The model under review builds one solid part; all positions refer to its coordinate system, in mm. A direction names the side the tool comes from. Round coordinates to 2 decimals unless told otherwise and drop trailing zeros. Write each loop counter-clockwise with the first axis right and the second up, starting at its lowest first coordinate (ties: lowest second). Pieces come first, ordered by that corner, then holes. Notation, with made-up numbers: (68, 29.5) -> (125, 29.5) arc R24 ccw to (125, 41.5) -> close; hole circle Ø6 at (76, -5). An arc over 180 degrees is marked (long way). Return JSON: item names as keys, results as strings. Group by question number.
1. Take a section at B-B, the plane x = -7.5. Write out the cut boundary in (y, z).
2. For line 1 along Z through (x, y) = (-7.3, -10.2); line 2 along X through (y, z) = (-70, 0.5); line 3 along Y through (x, z) = (-8.8, -10), list the stretches that pass through material, from the lowest coordinate up. Write a range as from..to.
3. Take a section at C-C, the plane y = -36. Write out the cut boundary in (x, z).
4. Clearance check with a flat-ended pin moving along its axis: P1, Ø14.5, axis at y = -78, z = 6.5, coming from the +X side. State where the tip first meets the part, or that it passes through.
5. Mouldability with a two-part tool opening along Y and no side actions: class faces 4 (the flat face through (-9.15, -127.44, 2.59)), 5 (the flat face through (-8, 0, -1)), 6 (the flat face through (-9, -50, 11.847)), 7 (the cylindrical face through (-8.083, -9.658, 3.207)) as pulls with the +Y half, pulls with the -Y half, needs draft (parallel to the pull), parting line crosses it, or undercut.
6. Take a section at A-A, the plane y = -10.2. Write out the cut boundary in (x, z).
7. Tool access review of faces 1 (the flat face through (-9.168, -66.634, -7.842)), 2 (the flat face through (-8, -16, -14.153)), 3 (the flat face through (-8.661, -81, 5)): name each direction out of +Z, -Z, +X, -X, +Y, -Y from which nothing blocks a thin tool from reaching the whole face with its end or side.
from build123d import *

# Parameters (mm, degrees)
F1_DEPTH = 31.5
F2_DEPTH = 131.5
F6_DEPTH = 25
F7_D     = 5
F7_DEPTH = 300
F7_START = 6.4609628
F7_TIP   = 1.5021515476


with BuildPart() as f1:
    # F0 (on Front) → F1 (new body)
    with BuildSketch(Plane.XZ):
        Polygon((-8.6609627543, 11.8473982275), (-9.6609627543, 11.8473982275), (-9.6609627543, -14.1526017725), (-8.6609627543, -1.3526017725), align=None)
        Polygon((-6.4609627543, 11.8473982275), (-8.6609627543, 11.8473982275), (-8.6609627543, -1.3526017725), (-9.6609627543, -14.1526017725), (-8.6609627543, -14.1526017725), (-6.4609627543, -14.1526017725), align=None)
    extrude(amount=F1_DEPTH)

    # F0 (on Front) → F2 (join)
    with BuildSketch(Plane.XZ):
        Polygon((-8.6609627543, 11.8473982275), (-9.6609627543, 11.8473982275), (-9.6609627543, -14.1526017725), (-8.6609627543, -1.3526017725), align=None)
    extrude(amount=F2_DEPTH)

    # F5 (on Right) → F6 (cut)
    with BuildSketch(Plane.YZ):
        Polygon((-123.5, -1.3526017725), (-131.5, -1.3526017725), (-131.5, -14.1526017725), (-123.5, -14.1526017725), (-91.8188882763, -14.1526017725), align=None)
        Polygon((-123.5, -1.3526017725), (-131.5, 6.6473982275), (-131.5, -1.3526017725), align=None)
    extrude(amount=-F6_DEPTH, mode=Mode.SUBTRACT)

    # F7
    # its depths count from where the whole tool has entered the part; down to there all is cleared
    with Locations(Plane.YZ.offset(-F7_START)):
        with Locations((-10.2, 5.6473982275), (-10.2, -8.3526017725)):
            Hole(F7_D / 2, depth=F7_DEPTH)
            with Locations((0, 0, -(F7_DEPTH + F7_TIP / 2))):  # 118° drill point
                Cone(0, F7_D / 2, F7_TIP, mode=Mode.SUBTRACT)


solid = f1.part
Output:
{
 "1": {"outline": "(-31.5, -14.15) -> (0, -14.15) -> (0, 11.85) -> (-31.5, 11.85) -> close; hole circle Ø5 at (-10.2, -8.35); hole circle Ø5 at (-10.2, 5.65)"},
 "2": {"line 1": "z = -14.15..-10.85, -5.85..3.15, 8.15..11.85", "line 2": "x = -9.66..-8.66", "line 3": "y = -31.5..-12.08, -8.32..0"},
 "3": {"outline": "(-9.66, -14.15) -> (-8.66, -1.35) -> (-8.66, 11.85) -> (-9.66, 11.85) -> close"},
 "4": {"P1": "stops at x = -8.66"},
 "5": {"face 4": "pulls with the -Y half", "face 5": "pulls with the +Y half", "face 6": "needs draft", "face 7": "undercut"},
 "6": {"outline": "(-9.66, -14.15) -> (-6.46, -14.15) -> (-6.46, -10.85) -> (-9.66, -10.85) -> close; (-9.66, -5.85) -> (-6.46, -5.85) -> (-6.46, 3.15) -> (-9.66, 3.15) -> close; (-9.66, 8.15) -> (-6.46, 8.15) -> (-6.46, 11.85) -> (-9.66, 11.85) -> close"},
 "7": {"face 1": "-Z, +X, -Y", "face 2": "-Z, +X, -X, +Y, -Y", "face 3": "+Z, -Z, +X, -Y"}
}
